```python
from build123d import *

# Parameters (mm, degrees)
SKETCH1_R                = 100
BOSS_EXTRUDE1_DEPTH      = 5
SKETCH4_R                = 3
CUT_EXTRUDE2_DEPTH       = 142.509716981
CIRPATTERN1_COUNT        = 6
M6_CLEARANCE_HOLE1_D     = 6.6
SKETCH7_W                = 14
SKETCH7_H                = 5
CUT_EXTRUDE3_DEPTH       = 142.509716981
SKETCH8_R                = 1
SKETCH8_R_2              = 3.1
CUT_EXTRUDE4_DEPTH       = 142.509716981
F_0000_CLEARANCE_HOLE3_D = 0.6604
FILLET1_R                = 0.5
SKETCH20_R               = 1.5
CUT_EXTRUDE6_DEPTH       = 142.509716981
SKETCH21_R               = 10
CUT_EXTRUDE9_DEPTH       = 142.509716981


with BuildPart() as part:
    # Sketch1 → Boss-Extrude1 (new body)
    with BuildSketch(Plane.XY):
        Circle(SKETCH1_R)
    extrude(amount=BOSS_EXTRUDE1_DEPTH)

    # Sketch4 → Cut-Extrude2 (cut, through all)
    with BuildSketch(Plane.XY):
        with Locations((0, 50)):
            Circle(SKETCH4_R)
    cut_extrude2 = extrude(amount=CUT_EXTRUDE2_DEPTH, mode=Mode.SUBTRACT)

    # CirPattern1: Cut-Extrude2 ×6 about axis
    cirpattern1_axis = Axis((0, 0, 0), (0, 0, 1))
    for i in range(1, CIRPATTERN1_COUNT):
        add(cut_extrude2.rotate(cirpattern1_axis, i * 360 / CIRPATTERN1_COUNT), mode=Mode.SUBTRACT)

    # M6 Clearance Hole1 (through all)
    with Locations(Plane.XY.offset(5)):
        with Locations((0, 50), (43.301270189, 25), (43.301270189, -25), (0, -50), (-43.301270189, -25), (-43.301270189, 25)):
            Hole(M6_CLEARANCE_HOLE1_D / 2)

    # Sketch7 → Cut-Extrude3 (cut, through all)
    with BuildSketch(Plane.XY):
        with Locations((2.5, -19.5)):
            Rectangle(SKETCH7_W, SKETCH7_H)
    extrude(amount=CUT_EXTRUDE3_DEPTH, mode=Mode.SUBTRACT)

    # Sketch8 → Cut-Extrude4 (cut, through all)
    with BuildSketch(Plane(origin=(0, 0, 0), x_dir=(-1, 0, 0), z_dir=(0, 0, -1))):
        with Locations((-2.5, 4)):
            Circle(SKETCH8_R)
        with Locations((-2.5, -17)):
            Circle(SKETCH8_R_2)
    extrude(amount=-CUT_EXTRUDE4_DEPTH, mode=Mode.SUBTRACT)

    # #0000 Clearance Hole3 (through all)
    with Locations(Plane(origin=(0, 0, 0), x_dir=(-1, 0, 0), z_dir=(0, 0, -1))):
        with Locations((-2.5, 4), (0, 0), (0, -100)):
            Hole(F_0000_CLEARANCE_HOLE3_D / 2)

    # Fillet1
    fillet1_edges = [part.edges().sort_by_distance(p)[0] for p in [
        (5.6, -17, 2.5),
        (-0.6, -17, 2.5),
    ]]
    fillet(fillet1_edges, radius=FILLET1_R)

    # Sketch20 → Cut-Extrude6 (cut, through all)
    with BuildSketch(Plane(origin=(0, 0, 0), x_dir=(-1, 0, 0), z_dir=(0, 0, -1))):
        with Locations((-8.5, -37)):
            Circle(SKETCH20_R)
        with Locations((3.5, -37)):
            Circle(SKETCH20_R)
    extrude(amount=-CUT_EXTRUDE6_DEPTH, mode=Mode.SUBTRACT)

    # Sketch21 → Cut-Extrude9 (cut, through all)
    with BuildSketch(Plane.XY):
        Circle(SKETCH21_R)
    extrude(amount=CUT_EXTRUDE9_DEPTH, mode=Mode.SUBTRACT)


solid = part.part
```
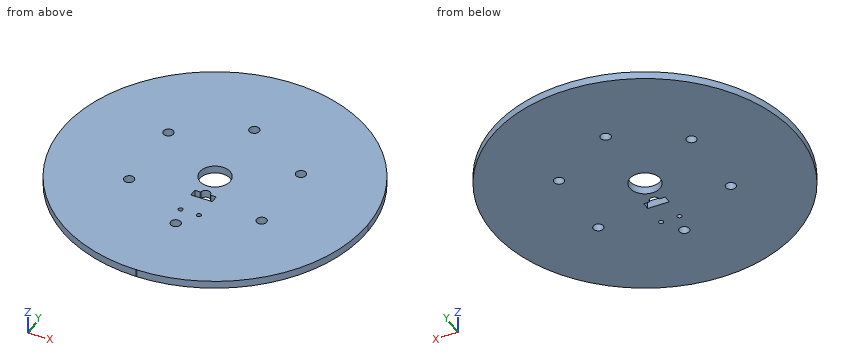
Geometry: final body of the model. Coordinates: model frame, mm. Give positions to 0.01 mm unless a question says otherwise; leave off trailing zeros. Write each loop counter-clockwise with the first axis right and the second up, starting at its lowest first coordinate (ties: lowest second). Pieces come first, ordered by that corner, then holes.
1. Section query C-C, the plane x = 44. Return loops of the section in (y, z), then the cut area to 3 significant figures.
2. Section query A-A, the plane y = -50. Return loops of the section in (x, z).
3. Line query: probe 1 along Y at (x, z) = (0, 2.8); probe 2 along Y at (x, z) = (-41.5, 0.85); probe 3 along Y at (x, z) = (-3.5, 1). Output: solid intervals per line, ascending.
4. Section query D-D, the plane y = -25. Return loops of the section in (x, z).
5. Section query B-B, the plane z = 3.7. Count the separate pieces of the cut face and the enclosed holes in it, then the cut area to 3 significant figures.
6. Pin query (flat end, axial travel): P1, Ø1.5, axis at x = 3, z = 2.5, coming from the +Y side; P2, Ø2.5, axis at x = -2, z = 1.5, coming from the -Y side; P3, Ø1.5, axis at y = -60, z = 4.5, coming from the -X side. Return the tip coordinate at first contact, or that it passes through.
Computed:
1. outline: (-89.8, 0) - (-28.23, 0) - (-28.23, 5) - (-89.8, 5) - close; (-21.77, 0) - (21.77, 0) - (21.77, 5) - (-21.77, 5) - close; (28.23, 0) - (89.8, 0) - (89.8, 5) - (28.23, 5) - close
1. area: 833 mm2
2. outline: (-86.6, 0) - (-3.3, 0) - (-3.3, 5) - (-86.6, 5) - close; (3.3, 0) - (86.6, 0) - (86.6, 5) - (3.3, 5) - close
3. probe 1: y = -99.67 to -53.3, -46.7 to -22, -15.17 to -10, 10 to 46.7, 53.3 to 100
3. probe 2: y = -90.98 to -27.77, -22.23 to 22.23, 27.77 to 90.98
3. probe 3: y = -99.94 to -38.5, -35.5 to -22, -17 to -9.37, 9.37 to 99.94
4. outline: (-96.82, 0) - (-46.6, 0) - (-46.6, 5) - (-96.82, 5) - close; (-40, 0) - (40, 0) - (40, 5) - (-40, 5) - close; (46.6, 0) - (96.82, 0) - (96.82, 5) - (46.6, 5) - close
5. separate pieces: 1
5. enclosed holes: 10
5. area: 30,800 mm2
6. P1: stops at y = 99.97
6. P2: stops at y = -100
6. P3: stops at x = -80.56
